```python
from build123d import *

# Parameters (mm, degrees)
SKETCH1_R           = 1.65
BOSS_EXTRUDE1_DEPTH = 3
BOSS_EXTRUDE2_DEPTH = 10


with BuildPart() as part:
    # Sketch1 → Boss-Extrude1 (new body)
    with BuildSketch(Plane(origin=(0, 0, 0), x_dir=(1, 0, 0), z_dir=(0, 1, 0))):
        Polygon((-3, 30.5), (-3, -3), (3, -3), (3, 30.5), (15.678547852, 57.689233611), (13.214366438, 58.838300276), (3, 36.933520762), (0.535818585, 38.082587426), align=None)
        with Locations(Location((0, 30.5, 0), (0, 0, 270))):
            Circle(SKETCH1_R, mode=Mode.SUBTRACT)
        with Locations(Location((0, 0, 0), (0, 0, 270))):
            Circle(SKETCH1_R, mode=Mode.SUBTRACT)
    extrude(amount=BOSS_EXTRUDE1_DEPTH)

    # Sketch1_4 → Boss-Extrude2 (add)
    with BuildSketch(Plane(origin=(0, 0, 0), x_dir=(1, 0, 0), z_dir=(0, 1, 0))):
        Polygon((10.750185023, 59.98736694), (0.535818585, 38.082587426), (3, 36.933520762), (13.214366438, 58.838300276), align=None)
    extrude(amount=BOSS_EXTRUDE2_DEPTH)


solid = part.part
```
Work out the finished part from the listing and answer in its coordinate system (mm). A direction names the side the tool comes from. Give positions to 0.01 mm unless a question says otherwise; leave off trailing zeros. Loops run counter-clockwise (first coordinate to the right, second up) from the corner with the lowest first, then second, coordinate; pieces in that order, holes last. Notation, with made-up numbers: (52, 15) -> (99, 15) arc R17 cw to (99, 42) -> close; hole circle Ø7 at (83.5, 83). An arc over 180 degrees is marked (long way). One line per question, with ' | ' between items. Start each with the question number.
1) Straight lines are drawn through the part: L1, parallel to X at y = 1.75, z = -30.5; L2, parallel to Y at x = 1, z = -19.5; L3, parallel to X at y = 7, z = -47.5. For each, find the intervals that lie inside material, in ascending order.
2) Each of these flat-tipped pins is pushed along its axis until it touches: pin 1 (1.5 mm diameter, centred on y = 1, z = -11, fed in from +X); pin 2 (4 mm diameter, centred on x = 0, z = 0, fed in from +Y); pin 3 (5 mm diameter, centred on x = 11, y = 1.5, fed in from +Z); pin 4 (4 mm diameter, centred on x = 0, z = -30.5, fed in from -Y). Where does it stop, or does it pass through?
3) Section C-C, the plane x = 7.5 is taken. Determine the outline of the cut face in (y, z), then the cut area to 3 significant figures.
4) Section A-A, the plane x = 0 is taken. Determine the outline of the cut face in (y, z).
5) Section B-B, the plane y = 8 is taken. Determine the outline of the cut face in (x, z), then the cut area to 3 significant figures.
6) Determine the mould class of faces 1 (the face through (1.751, 6.451, -37.516)), 2 (the face through (-3, 1, -14)), 3 (the face through (-1, 1.48, -1.31)) for opening direction Z: +Z half, -Z half, draft (parallel to the pull), parting line (faces both ways), or undercut.
7) Section D-D, the plane z = -35 is taken. Determine the outline of the cut face in (x, y).
8) For faces 4 (the face through (8.036, 6.451, -47.733)), 5 (the face through (3, 1, -14)), 6 (the face through (2.8, 0, -28.6)), determine the directions among +Z, -Z, +X, -X, +Y, -Y from which every point of the face is accessible in a straight line to the end or side of a thin tool.
Resolved:
1) L1: -3 to -1.65, 1.65 to 3 | L2: 0 to 3 | L3: 4.93 to 7.93
2) pin 1: x = 3 | pin 2: y = 3 | pin 3: z = -42.29 | pin 4: y = 0
3) outline: (0, -53.02) -> (10, -53.02) -> (10, -46.58) -> (3, -46.58) -> (3, -40.15) -> (0, -40.15) -> close | area: 83.6 mm2
4) outline: (0, -36.93) -> (3, -36.93) -> (3, -32.15) -> (0, -32.15) -> close; (0, -28.85) -> (3, -28.85) -> (3, -1.65) -> (0, -1.65) -> close; (0, 1.65) -> (3, 1.65) -> (3, 3) -> (0, 3) -> close
5) outline: (0.54, -38.08) -> (10.75, -59.99) -> (13.21, -58.84) -> (3, -36.93) -> close | area: 65.7 mm2
6) face 1: +Z half | face 2: draft | face 3: undercut
7) outline: (-0.9, 0) -> (5.1, 0) -> (5.1, 3) -> (-0.9, 3) -> close
8) face 4: +Z, +X, +Y | face 5: +Z, +X, +Y, -Y | face 6: +Z, -Z, +X, -X, -Y
